```python
from build123d import *

# Parameters (mm, degrees)
CONG_1_R = 0.15


with BuildPart() as part:
    # Esquisse1 → Base-Révolution (revolve)
    with BuildSketch(Plane.XY):
        with BuildLine():
            Line((0, 1.5), (0, 2.5))
            Line((0, 2.5), (1, 2.5))
            ThreePointArc((1, 2.5), (2, 2), (3, 2.5))
            Line((3, 2.5), (4, 2.5))
            Line((4, 2.5), (4, 1.5))
            Line((4, 1.5), (0, 1.5))
        make_face()
    revolve(axis=Axis((0, 0, 0), (1, 0, 0)))

    # Congé1
    cong_1_edges = [part.edges().sort_by_distance(p)[0] for p in [
        (0, -1.5, 0),
        (4, -1.5, 0),
    ]]
    fillet(cong_1_edges, radius=CONG_1_R)


solid = part.part
```
Here's how the part is built. I have some questions about the finished solid (model axes, mm). Give positions to 0.01 mm unless a question says otherwise; leave off trailing zeros. Loops run counter-clockwise (first coordinate to the right, second up) from the corner with the lowest first, then second, coordinate; pieces in that order, holes last. Notation, with made-up numbers: M -6.5,36.25 L 4.5,36.25 A27 ccw 4.5,53.25 Z; hole C 52.5,33 d6. An arc over 180 degrees is marked long. Put each result on its own line as item: value. Start each with the question number.
(1) I want a section at D-D on x = 1.55. Please give me the cut outline in (y, z), then the cut area to 3 significant figures.
(2) If we mould it in two halves opening along Z, with no side actions, what happens to faces 1 (the cylindrical face through (1.97, -1.5, 0.07)), 2 (the cylindrical face through (3.51, -0.54, -2.44)), 3 (the flat face through (4, 2, -1))? For each: +Z half, -Z half, draft (parallel to the pull), parting line (faces both ways), or undercut.
(3) Will these pins go through, and if not, where does the flat tip stop? pin 1 Ø1.5 at (x, z) = (1.5, 0) entering from -Y; pin 2 Ø1 at (x, z) = (2, -0.5) entering from -Y.
(4) I want a section at C-C on x = 3.55. Please give me the cut outline in (y, z), then the cut area to 3 significant figures.
(5) I want a section at A-A on y = 0. Please give me the cut outline in (x, z).
(6) I need wall thicknesses on line 1 along Z through (x, y) = (3.1, 0); line 2 along X through (y, z) = (-0.4, 2.25); line 3 along Z through (x, y) = (1.4, -0.75). Which ranges of each line are inside material? Lowest first, please. Write a range as [from, to].
Answer block:
1. outline: C 0,0 d4.17; hole C 0,0 d3
1. area: 6.57 mm^2
2. face 1: undercut
2. face 2: parting line
2. face 3: draft
3. pin 1: y = -2.5
3. pin 2: y = -2.07
4. outline: C 0,0 d5; hole C 0,0 d3
4. area: 12.6 mm^2
5. outline: M 0,-2.5 L 1,-2.5 A1.25 cw 3,-2.5 L 4,-2.5 L 4,-1.65 A0.15 ccw 3.85,-1.5 L 0.15,-1.5 A0.15 ccw 0,-1.65 Z; M 0,1.65 A0.15 ccw 0.15,1.5 L 3.85,1.5 A0.15 ccw 4,1.65 L 4,2.5 L 3,2.5 A1.25 cw 1,2.5 L 0,2.5 Z
6. line 1: [-2.5, -1.5], [1.5, 2.5]
6. line 2: [0, 1.21], [2.79, 4]
6. line 3: [-2.02, -1.3], [1.3, 2.02]
